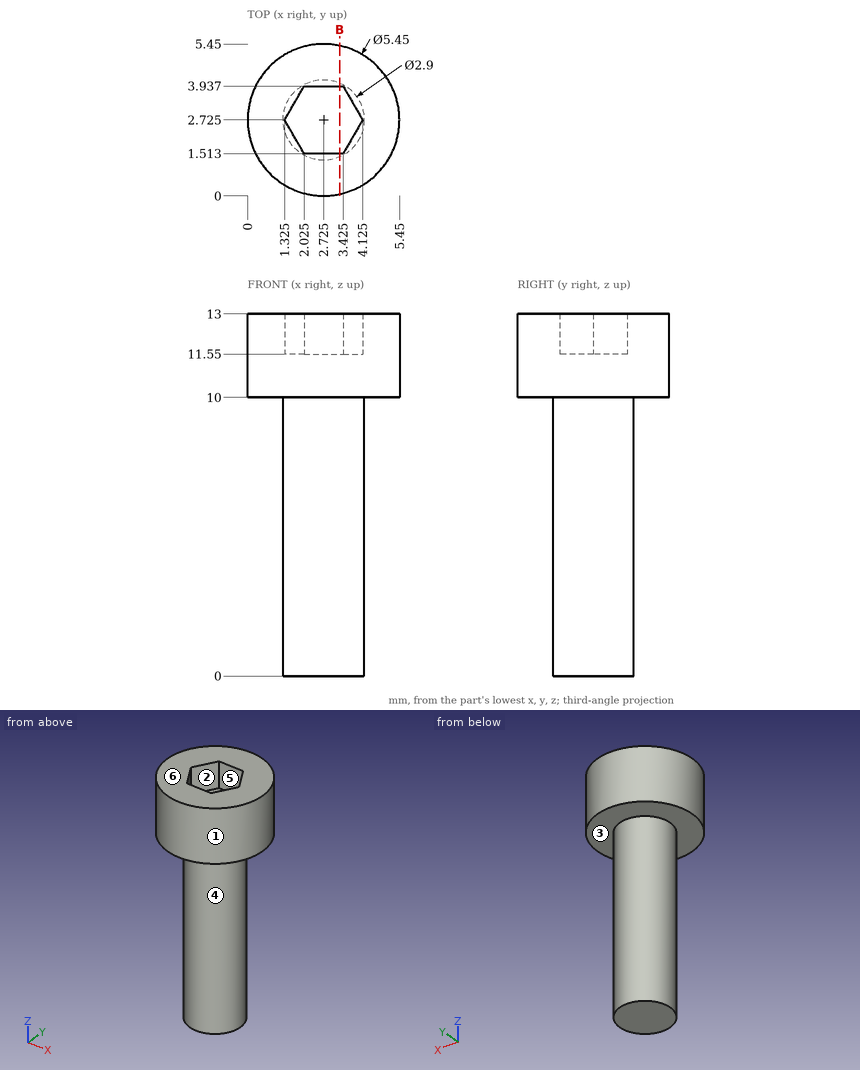
Drawing for the job (mm, zero at the part's lowest x, y, z). A direction names the side the tool comes from. Give positions to 0.01 mm unless a question says otherwise; leave off trailing zeros. Order: outer loops, then holes, each group sorted by start corner. A loop starts at its lowest first (then second) coordinate and runs counter-clockwise, first axis right, second up. Notation, with made-up numbers: M 17,-21.75 L 65,-21.75 A13 ccw 65,-8.75 Z; hole C 40,-35.75 d2. An arc over 180 degrees is marked long. Use a Markdown table: item, result. Add a question column.
(1) Mould opens along X. For the marked faces 1, 2 and 3 say: +X half, -X half, draft (parallel to the pull), parting line (faces both ways), or undercut.
(2) Drop flat-ended pins along their axis: P1, Ø3, axis at x = 4, z = 4, coming from the +Y side (3 decimals); P2, Ø1.2, axis at x = 3.5, y = 3, coming from the +Z side; P3, Ø1, axis at y = 5, z = 6, coming from the +X side; P4, Ø2, axis at x = 4.5, z = 8, coming from the +Y side. Give the stop position or say it passes through.
(3) Saw through at B-B, the plane x = 3.3. Give the cut face in (y, z).
(4) 3-axis set-ups, long thin cutter, end or side, ignore diameter. For the marked faces 4, 5 and 6: which of +Z, -Z, +X, -X, +Y, -Y reach the whole face in a straight line?
(5) Probe line 1 along Z through (x, y) = (0.7, 2.2); line 2 along Z through (x, y) = (1.95, 3.35); line 3 along X through (y, z) = (2.25, 11.75). List the from-to ranges inside material, lowest first. Write a range as [from, to].
Answer key:
| question | item | result |
|---|---|---|
| 1 | face 1 | parting line |
| 1 | face 2 | undercut |
| 1 | face 3 | draft |
| 2 | P1 | y = 4.175 |
| 2 | P2 | z = 13 |
| 2 | P3 | through |
| 2 | P4 | y = 3.95 |
| 3 | outline | M 0.06,10 L 1.39,10 L 1.39,0 L 4.06,0 L 4.06,10 L 5.39,10 L 5.39,13 L 3.94,13 L 3.94,11.55 L 1.51,11.55 L 1.51,13 L 0.06,13 Z |
| 4 | face 4 | -Z |
| 4 | face 5 | +Z |
| 4 | face 6 | +Z, +X, -X, +Y, -Y |
| 5 | line 1 | [10, 13] |
| 5 | line 2 | [0, 11.55] |
| 5 | line 3 | [0.04, 1.6], [3.85, 5.41] |
